Check sheet for the modelled part. Datum: model origin and axes. Units: mm. A direction names the side the tool comes from. Give positions to 0.01 mm unless a question says otherwise; leave off trailing zeros. Loops run counter-clockwise (first coordinate to the right, second up) from the corner with the lowest first, then second, coordinate; pieces in that order, holes last. Notation, with made-up numbers: M -26.5,69.5 L 12.5,69.5 A35 ccw 12.5,104.5 Z; hole C 39.25,35 d10. An arc over 180 degrees is marked long. Put each result on its own line as item: value. Start each with the question number.
```python
from build123d import *

# Parameters (mm, degrees)
SKETCH1_W            = 6.1468
SKETCH1_H            = 6.1468
BOSS_EXTRUDE1_DEPTH  = 3.7084
SKETCH2_R            = 1.7653
BOSS_EXTRUDE2_DEPTH  = 5.6134
BOSS_EXTRUDE3_DEPTH  = 0.635
MIRROR2_COPY_1_DEPTH = 0.635


with BuildPart() as part:
    # Sketch1 → Boss-Extrude1 (new body)
    with BuildSketch(Plane.XY):
        Rectangle(SKETCH1_W, SKETCH1_H)
    extrude(amount=BOSS_EXTRUDE1_DEPTH)

    # Sketch2 → Boss-Extrude2 (add)
    with BuildSketch(Plane.XY.offset(3.7084)):
        Circle(SKETCH2_R)
    extrude(amount=BOSS_EXTRUDE2_DEPTH)

    # Sketch3 → Boss-Extrude3 (add)
    with BuildSketch(Plane.ZY.offset(3.0734)):
        Polygon((1.8542, 3.0734), (1.8542, 3.355054083), (-0.299045368, 3.8354), (-2.4638, 3.409917683), (-2.4638, 3.0734), (-0.303331796, 3.49803982), (1.6002, 3.0734), align=None)
    boss_extrude3 = extrude(amount=-BOSS_EXTRUDE3_DEPTH)

    # Mirror1: Boss-Extrude3 across plane
    add(boss_extrude3.mirror(Plane.ZY))

    # Mirror2: Boss-Extrude3 across plane
    add(boss_extrude3.mirror(Plane.ZX))

    # Mirror2 copy 1 sketch → Mirror2 copy 1 (add)
    with BuildSketch(Plane(origin=(3.0734, 0, 0), x_dir=(0, 0, 1), z_dir=(1, 0, 0))):
        Polygon((1.8542, 3.0734), (1.8542, 3.355054083), (-0.299045368, 3.8354), (-2.4638, 3.409917683), (-2.4638, 3.0734), (-0.303331796, 3.49803982), (1.6002, 3.0734), align=None)
    extrude(amount=-MIRROR2_COPY_1_DEPTH)


solid = part.part
```
Q1. Depth check by flat-ended pin: P1, Ø1, axis at x = -1, z = 3.5, coming from the +Y side; P2, Ø1, axis at y = -1, z = 7.5, coming from the +X side; P3, Ø3, axis at x = 1, y = 1, coming from the -Z side. Enter the tip coordinate at first touch or a pass-through.
Q2. Section check D-D, the plane z = 0.5. Record the cut outline in (x, y).
Q3. Section check B-B, the plane z = -1. Record the cut outline in (x, y).
Q4. Thickness scan on line 1 along Z through (x, y) = (-1.5, 1.5); line 2 along Y through (x, z) = (2.25, 1.5); line 3 along Z through (x, y) = (-1.25, 0.75). Record the ranges inside material, lowest first. Write a range as [from, to].
Q5. Access from +Z, -Z, +X, -X, +Y, -Y to the whole of each face (thin tool, end or side, straight path). Record for faces 1 (the face through (0, 0, 0)), 2 (the face through (3.073, 0, 1)), 3 (the face through (0.81, -1.57, 6.48)).
Q6. Section check A-A, the plane x = 0. Record the cut outline in (y, z).
Found:
1. P1: stops at y = 3.07
1. P2: stops at x = 1.69
1. P3: stops at z = 0
2. outline: M -3.07,-3.66 L -2.44,-3.66 L -2.44,-3.32 L -3.07,-3.32 Z; M -3.07,-3.07 L 3.07,-3.07 L 3.07,3.07 L -3.07,3.07 Z; M -3.07,3.32 L -2.44,3.32 L -2.44,3.66 L -3.07,3.66 Z; M 2.44,-3.66 L 3.07,-3.66 L 3.07,-3.32 L 2.44,-3.32 Z; M 2.44,3.32 L 3.07,3.32 L 3.07,3.66 L 2.44,3.66 Z
3. outline: M -3.07,-3.7 L -2.44,-3.7 L -2.44,-3.36 L -3.07,-3.36 Z; M -3.07,3.36 L -2.44,3.36 L -2.44,3.7 L -3.07,3.7 Z; M 2.44,-3.7 L 3.07,-3.7 L 3.07,-3.36 L 2.44,-3.36 Z; M 2.44,3.36 L 3.07,3.36 L 3.07,3.7 L 2.44,3.7 Z
4. line 1: z = [0, 3.71]
4. line 2: y = [-3.07, 3.07]
4. line 3: z = [0, 9.32]
5. face 1: -Z, +X, -X
5. face 2: +Z, -Z, +X, +Y, -Y
5. face 3: +Z
6. outline: M -3.07,0 L 3.07,0 L 3.07,3.71 L 1.77,3.71 L 1.77,9.32 L -1.77,9.32 L -1.77,3.71 L -3.07,3.71 Z
